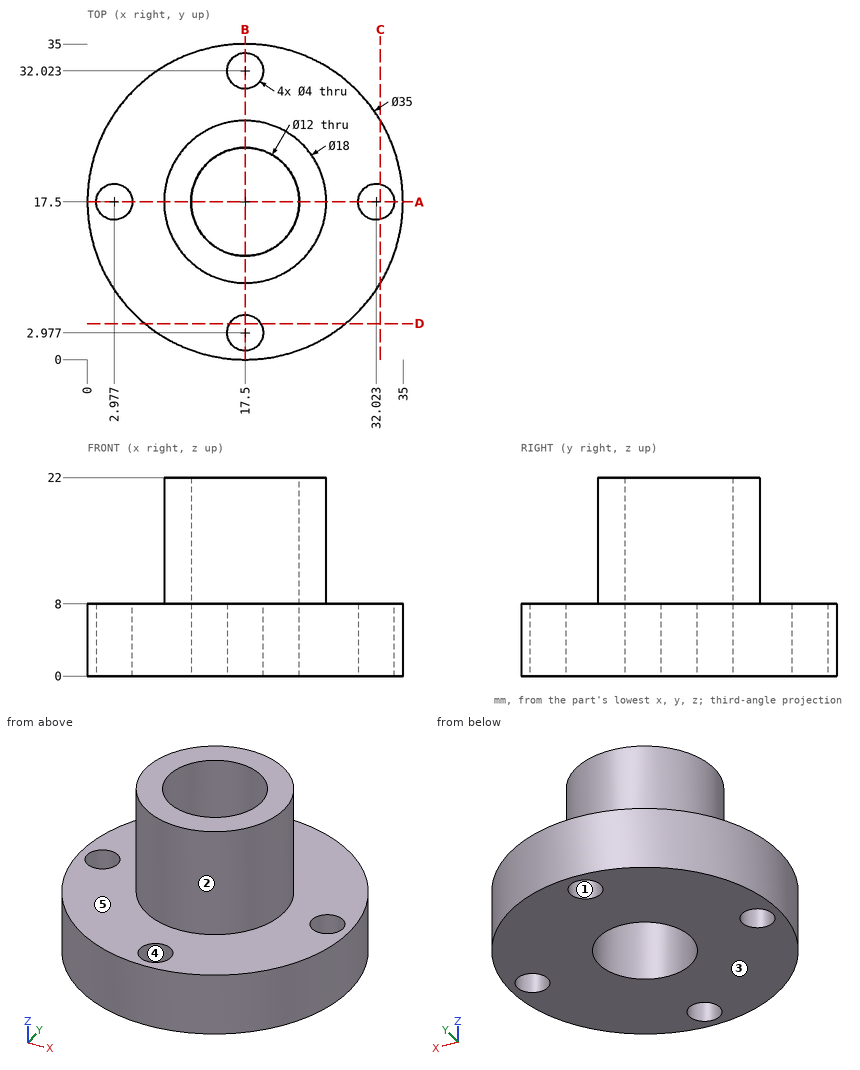
Verification items for this drawing (mm, ordinates from the low corner). A direction names the side the tool comes from. Give positions to 0.01 mm unless a question says otherwise; leave off trailing zeros. Loops run counter-clockwise (first coordinate to the right, second up) from the corner with the lowest first, then second, coordinate; pieces in that order, holes last.
1. Cross-section at A-A on y = 17.5. Record the cut outline in (x, z), and give its area (3 significant figures).
Derived:
outline: (0, 0) - (0.98, 0) - (0.98, 8) - (0, 8) - close; (4.98, 0) - (11.5, 0) - (11.5, 22) - (8.5, 22) - (8.5, 8) - (4.98, 8) - close; (23.5, 0) - (30.02, 0) - (30.02, 8) - (26.5, 8) - (26.5, 22) - (23.5, 22) - close; (34.02, 0) - (35, 0) - (35, 8) - (34.02, 8) - close
area: 204 mm2
2. Cross-section at C-C on x = 32.5. Record the cut outline in (y, z).
Derived:
outline: (8.49, 0) - (15.56, 0) - (15.56, 8) - (8.49, 8) - close; (19.44, 0) - (26.51, 0) - (26.51, 8) - (19.44, 8) - close
3. Tool access check on the marked faces 4 and 5. Record the directions out of +Z, -Z, +X, -X, +Y, -Y that give a thin tool (end or side, any length) a straight path to the whole face; none if there is none.
Derived:
face 4: +Z, -Z
face 5: +Z
4. Release check for a two-part mould opening along X. For the marked faces 1, 2 and 3 record: +X half, -X half, draft (parallel to the pull), parting line (faces both ways), or undercut.
Derived:
face 1: undercut
face 2: parting line
face 3: draft
5. Cross-section at D-D on y = 4. Record the cut outline in (x, z), and give its area (3 significant figures).
Derived:
outline: (6.36, 0) - (15.78, 0) - (15.78, 8) - (6.36, 8) - close; (19.22, 0) - (28.64, 0) - (28.64, 8) - (19.22, 8) - close
area: 151 mm2
6. Material ranges on probe 1 along Y at (x, z) = (17.5, 3.25); probe 2 along Y at (x, z) = (17.5, 15.75); probe 3 along Z at (x, y) = (30.5, 24.5), recorded low to high.
Derived:
probe 1: y = 0 to 0.98, 4.98 to 11.5, 23.5 to 30.02, 34.02 to 35
probe 2: y = 8.5 to 11.5, 23.5 to 26.5
probe 3: z = 0 to 8
7. Go/stop test with flat-tipped pins: P1, Ø2.5, axis at x = 17.5, y = 32.02, coming from the +Z side; P2, Ø1, axis at y = 16.5, z = 13.5, coming from the -X side; P3, Ø10, axis at x = 24, z = 14.5, coming from the -Y side; P4, Ø3, axis at x = 15.5, z = 9, coming from the -Y side. Record where each tip stops, or that it passes through.
Derived:
P1: passes through
P2: stops at x = 8.51
P3: stops at y = 8.63
P4: stops at y = 0.02
